```python
from build123d import *

# Parameters (mm, degrees)
F0_W     = 40
F0_H     = 24.5
F1_DEPTH = 8
F2_T     = -2
F3_R     = 1
F4_DEPTH = 25
F5_R     = 1.99999
F7_DEPTH = 22.5


# Not quite as in the source:
# - a fillet or chamfer is up to 0.001 mm smaller than in the source, because OpenCascade refuses the exact size


with BuildPart() as f1:
    # F0 (on Top) → F1 (new body)
    with BuildSketch(Plane.XY):
        Rectangle(F0_W, F0_H)
    extrude(amount=F1_DEPTH)

    # F2
    f2_openings = [f1.faces().sort_by_distance(p)[0] for p in [
        (0, 0, 0),
    ]]
    offset(amount=F2_T, openings=f2_openings)

    # F3 (on face) → F4 (cut)
    with BuildSketch(Plane.XZ.offset(12.25)):
        with Locations((17, 3)):
            Circle(F3_R)
        with BuildLine():
            ThreePointArc((17, 6), (19.1213203436, 5.1213203436), (20, 3))
            Line((20, 3), (20, 8))
            Line((20, 8), (14, 8))
            Line((14, 8), (14, 6))
            Line((14, 6), (17, 6))
        make_face()
        with BuildLine():
            ThreePointArc((20, 3), (19.1213203436, 0.8786796564), (17, 0))
            Line((17, 0), (20, 0))
            Line((20, 0), (20, 3))
        make_face()
    extrude(amount=-F4_DEPTH, mode=Mode.SUBTRACT)

    # F5 (radius 2 in the source; OpenCascade refuses exactly that, so slightly less here)
    f5_edges = [f1.edges().sort_by_distance(p)[0] for p in [
        (-20, 0, 8),
        (14, 0, 8),
    ]]
    fillet(f5_edges, radius=F5_R)

    # F6 (on face) → F7 (join)
    with BuildSketch(Plane.XZ.offset(-10.25)):
        with BuildLine():
            Line((14, 6), (13.095, 6))
            Line((13.095, 6), (13.095, 4.4142135624))
            Line((13.095, 4.4142135624), (18, 4.4142135624))
            Line((18, 4.4142135624), (18, 5.8284271247))
            ThreePointArc((18, 5.8284271247), (17.5073059362, 5.956795679), (17, 6))
            Line((17, 6), (14, 6))
        make_face()
    extrude(amount=F7_DEPTH)


solid = f1.part
```
Design review of the part built by this model. Coordinates are the model's own, in mm. A direction names the side the tool comes from. Coordinates: 2 decimals unless noted, no trailing zeros. Loops run counter-clockwise (first coordinate to the right, second up) from the corner with the lowest first, then second, coordinate; pieces in that order, holes last. Notation, with made-up numbers: M 24.25,80 L 57.25,80 A13 cw 57.25,98 Z; hole C -37,24.5 d9. An arc over 180 degrees is marked long. One line per question, with ' | ' between items.
(1) Draft analysis for pull direction X (two halves, no side actions). For faces 1 (the face through (0, 12.25, 4)), 2 (the face through (18, 11, 3)), 3 (the face through (-19.43, 0.17, 7.4)), state which applies: released by +X, released by -X, zero draft, split by the parting line, or undercut.
Filled in:
face 1: zero draft | face 2: undercut | face 3: released by -X
(2) Wall thickness on probe 1 along Y at (x, z) = (0, 5); probe 2 along Z at (x, y) = (17, 11.3); probe 3 along Z at (x, y) = (16, 1.5): over which ranges is each line inside the solid? List them lowest first.
Filled in:
probe 1: y = -12.25 to -10.25, 10.25 to 12.25 | probe 2: z = 0 to 2, 4 to 6 | probe 3: z = 4.41 to 6
(3) We need section D-D (z = 0.75). Give the boundary of the cut face in (x, y), and give its area (3 significant figures).
Filled in:
outline: M -20,-12.25 L 18.98,-12.25 L 18.98,12.25 L -20,12.25 Z; hole M -18,-10.25 L 18,-10.25 L 18,10.25 L -18,10.25 Z | area: 217 mm^2
(4) For pin 1 Ø2 at (x, y) = (-16, -2.5) entering from -Z; pin 2 Ø3.5 at (x, y) = (15.5, 1.5) entering from +Z, all flat-tipped, find the tip position at first contact; note any pin that passes through.
Filled in:
pin 1: stops at z = 6 | pin 2: stops at z = 6.97
(5) Machinability: for faces 4 (the face through (15, 0, 6)), 5 (the face through (18, 0, 2)), 6 (the face through (-3, 0, 8)), which of the approach directions +Z, -Z, +X, -X, +Y, -Y give a long, thin tool a straight path to every point of the face, cutting with its end or side? Answer none if there is none.
Filled in:
face 4: +Z, +X, +Y, -Y | face 5: -Z | face 6: +Z, +X, -X, +Y, -Y
(6) We need section C-C (x = -1). Give the boundary of the cut face in (y, z).
Filled in:
outline: M -12.25,0 L -10.25,0 L -10.25,6 L 10.25,6 L 10.25,0 L 12.25,0 L 12.25,8 L -12.25,8 Z
(7) We need section A-A (z = 3.5). Give the boundary of the cut face in (x, y), and give its area (3 significant figures).
Filled in:
outline: M -20,-12.25 L 16.13,-12.25 L 16.13,-10.25 L -18,-10.25 L -18,10.25 L 16.13,10.25 L 16.13,12.25 L -20,12.25 Z; M 17.87,-12.25 L 19.96,-12.25 L 19.96,12.25 L 17.87,12.25 L 17.87,10.25 L 18,10.25 L 18,-10.25 L 17.87,-10.25 Z | area: 234 mm^2
